The listing builds one solid part. Answer for the finished solid, in the listing's coordinates (mm). Coordinates: 2 decimals unless noted, no trailing zeros. Order: outer loops, then holes, each group sorted by start corner. A loop starts at its lowest first (then second) coordinate and runs counter-clockwise, first axis right, second up. Notation, with made-up numbers: (25.5, 58) - (44.5, 58) arc R19 ccw to (44.5, 91) - close; hole circle Ø2 at (-31.5, 38). An arc over 180 degrees is marked (long way). Use one line per item in the form item = value. Start each with the question number.
Item 1: Consider line 1 along Y through (x, z) = (0, -150.25); line 2 along Z through (x, y) = (-1.5, 0); line 3 along Z through (x, y) = (-3.25, 0). Determine where each line is inside the solid, lowest interval first. Write a range as [from, to].
Item 2: Section B-B, the plane y = 0 is taken. Write down the section's boundary in (x, z).
Item 3: Section D-D, the plane z = 150 is taken. Write down the section's boundary in (x, y), and give its area (3 significant figures).
Item 4: Each of these flat-tipped pins is pushed along its axis until it touches: pin 1 Ø5 at (y, z) = (4, 15) entering from +X; pin 2 Ø3 at (x, z) = (6, 98) entering from -Y; pin 3 Ø2 at (x, z) = (3, 53) entering from +Y. Where does it stop, or does it pass through?
Item 5: Section A-A, the plane x = 0 is taken. Write down the section's boundary in (y, z).
Item 6: Section C-C, the plane z = -64.5 is taken. Write down the section's boundary in (x, y), and give its area (3 significant figures).
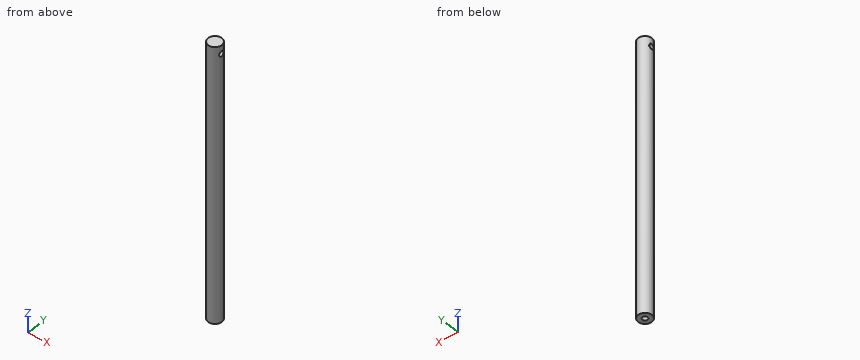
Autodesk Inventor part; units mm, degrees
ref_plane "YZ Plane" through (0, 0, 0) normal (1, 0, 0) x (0, 1, 0)
ref_plane "XZ Plane" through (0, 0, 0) normal (0, 1, 0) x (-1, 0, 0)
ref_plane "XY Plane" through (0, 0, 0) normal (0, 0, 1) x (1, 0, 0)
sketch "Skizze1" plane through (0, 0, 0) normal (0, 0, 1) x (1, 0, 0)
  circle A0 centre (0, 0) radius 8
  dimension "d0" = 16
extrude "Extrusion1" add sketch "Skizze1" along normal mid plane 320
sketch "Skizze6" plane through (0, 0, 0) normal (1, 0, 0) x (0, 1, 0)
  circle A0 centre (0, 150) radius 3
  line L0 (-4.2, 0) -> (4.2, 0)
  point P0 (0, 0)
  dimension "d16" = 6
  dimension "d19" = 150
extrude "Extrusion4" cut sketch "Skizze6" along normal mid plane 16
sketch "Skizze7" plane through (0, 0, -160) normal (0, 0, -1) x (-1, 0, 0)
  circle A0 centre (0, 0) radius 3
  dimension "d20" = 6
extrude "Extrusion5" cut sketch "Skizze7" against normal blind 30
thread "Gewinde2"
properties part number "Hauptpfeiler"
Response:
q1.line_1 = [-8, -3], [3, 8]
q1.line_2 = [-130, 147], [153, 160]
q1.line_3 = [-160, 147], [153, 160]
q2.outline = (-8, -160) - (-3, -160) - (-3, -130) - (3, -130) - (3, -160) - (8, -160) - (8, 147) - (-8, 147) - close; (-8, 153) - (8, 153) - (8, 160) - (-8, 160) - close
q3.outline = (-7.42, -3) arc R8 ccw to (7.42, -3) - close; (-7.42, 3) - (7.42, 3) arc R8 ccw to start
q3.area = 107 mm2
q4.pin_1 = 7.86
q4.pin_2 = -6.61
q4.pin_3 = 7.75
q5.outline = (-8, -160) - (-3, -160) - (-3, -130) - (3, -130) - (3, -160) - (8, -160) - (8, 160) - (-8, 160) - close; hole circle Ø6 at (0, 150)
q6.outline = circle Ø16 at (0, 0)
q6.area = 201 mm2
